For this review, use the dimensioned drawing (mm, ordinates from the lowest corner) and the shaded views. Round coordinates to 2 decimals unless told otherwise and drop trailing zeros. Order: outer loops, then holes, each group sorted by start corner. A loop starts at its lowest first (then second) coordinate and runs counter-clockwise, first axis right, second up. Notation, with made-up numbers: (51, 55.5) - (101, 55.5) arc R16 ccw to (101, 76.5) - close; hole circle Ø11 at (-30, 59). An arc over 180 degrees is marked (long way). Write item = value, one per line.
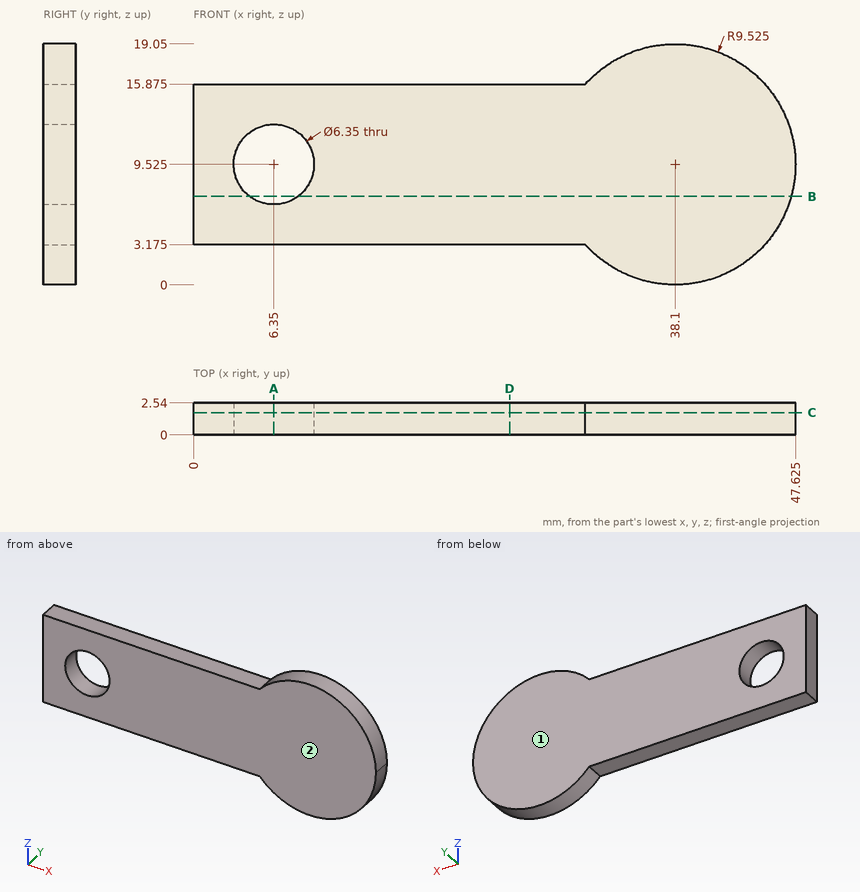
1) We need section C-C on y = 1.75. Write out the cut boundary in (x, z) (3 decimals), and give its area (3 significant figures).
Findings:
outline = (0, 3.175) - (31, 3.175) arc R9.525 ccw (long way) to (31, 15.875) - (0, 15.875) - close; hole circle Ø6.35 at (6.35, 9.525)
area = 626 mm^2
2) We need section B-B on z = 7. Write out the cut boundary in (x, y).
Findings:
outline = (0, 0) - (4.43, 0) - (4.43, 2.54) - (0, 2.54) - close; (8.27, 0) - (47.28, 0) - (47.28, 2.54) - (8.27, 2.54) - close
3) To check wall thickness, follow L1, parallel to Z at x = 9, y = 0.75 (3 decimals); L2, parallel to X at y = 1.4, z = 11.25; L3, parallel to Z at x = 6, y = 0.2 (3 decimals). State the ranges of each line that lie inside material, in increasing order. Write a range as from..to.
Findings:
L1 = 3.175..7.776, 11.274..15.875
L2 = 0..3.68, 9.02..47.47
L3 = 3.175..6.369, 12.681..15.875
4) We need section A-A on x = 6.35. Write out the cut boundary in (y, z) (3 decimals), and give its area (3 significant figures).
Findings:
outline = (0, 3.175) - (2.54, 3.175) - (2.54, 6.35) - (0, 6.35) - close; (0, 12.7) - (2.54, 12.7) - (2.54, 15.875) - (0, 15.875) - close
area = 16.1 mm^2
5) The part is to be moulded in two halves that separate along Y. For the marked faces 1 and 2, say which applies: released by +Y, released by -Y, zero draft, split by the parting line, or undercut.
Findings:
face_1 = released by +Y
face_2 = released by -Y
6) We need section D-D on x = 25. Write out the cut boundary in (y, z) (3 decimals).
Findings:
outline = (0, 3.175) - (2.54, 3.175) - (2.54, 15.875) - (0, 15.875) - close
7) Clearance check with flat-ended pins moving along their axes: pin 1 Ø1.3 at (x, y) = (14, 1.5) entering from +Z (3 decimals); pin 2 Ø1.3 at (x, y) = (9.5, 2) entering from -Z (3 decimals). State where each tip first meets the part, or that it passes through.
Findings:
pin_1 = 15.875
pin_2 = 3.175
